For this review, take the finished solid that the model builds, in its own axes (mm). A direction names the side the tool comes from. Coordinates: 2 decimals unless noted, no trailing zeros. Order: outer loops, then holes, each group sorted by start corner. A loop starts at its lowest first (then second) coordinate and runs counter-clockwise, first axis right, second up. Notation, with made-up numbers: (-31.5, -5.75) - (17.5, -5.75) arc R15 cw to (17.5, 2.25) - close; hole circle Ø4 at (30, 14). An arc over 180 degrees is marked (long way). One line per item, written item: value. Start each with the question number.
(1) To check wall thickness, follow line 1 along Z through (x, y) = (0, 1.25); line 2 along Y through (x, z) = (4, -5.5); line 3 along Y through (x, z) = (13, -10.5). State the ranges of each line that lie inside material, in increasing order.
(2) Clearance check with flat-ended pins moving along their axes: pin 1 (4 mm diameter, centred on x = 8.5, y = 20.5, fed in from -Z); pin 2 (3 mm diameter, centred on x = -19.5, z = 7.5, fed in from +Y); pin 3 (5 mm diameter, centred on y = 21.5, z = 7, fed in from -X); pin 4 (12 mm diameter, centred on x = 5.5, y = 9, fed in from +Z). State where each tip first meets the part, or that it passes through.
(3) Consider section D-D on y = 28.5. Write out the cut boundary in (x, z), then the cut area to 3 significant figures.
(4) Mouldability with a two-part tool opening along X and no side actions: class faces 4 (the flat face through (0, 35, 0)), 5 (the conical face through (0.13, 5.35, 14.54)), 6 (the cylindrical face through (-2.343, 33.493, 17.847)) as released by +X, released by -X, zero draft, split by the parting line, or undercut.
(5) For faces 1 (the cylindrical face through (0.71, 1.72, -19.21)), 2 (the cylindrical face through (-2.85, 4.49, 17.13)), 3 (the flat face through (0, 0, 0)), list the 3-axis set-ups (+Z, -Z, +X, -X, +Y, -Y) from which the entire face can be reached by the end or side of a thin tool; tool diameter is ignored.
(6) Consider section C-C on y = 12.5. Write out the cut boundary in (x, z).
(7) Consider section B-B on x = 0. Count the separate pieces of the cut face and the enclosed holes in it, then the cut area to 3 significant figures.
Autodesk Inventor part; units mm, degrees
ref_plane "YZ Plane" through (0, 0, 0) normal (1, 0, 0) x (0, 1, 0)
ref_plane "XZ Plane" through (0, 0, 0) normal (0, 1, 0) x (-1, 0, 0)
ref_plane "XY Plane" through (0, 0, 0) normal (0, 0, 1) x (1, 0, 0)
sketch "Sketch2" plane through (0, 0, 0) normal (0, 0, 1) x (1, 0, 0)
  line L0 (0, 0) -> (25, 0)
  line L1 (0, 0) -> (0, 35)
  line L2 (0, 35) -> (18, 35)
  line L3 (18, 35) -> (18, 30)
  line L4 (18, 30) -> (5, 30)
  line L5 (5, 30) -> (5, 7)
  line L6 (5, 7) -> (25, 7)
  line L7 (25, 7) -> (25, 0)
  dimension "d3" = 25
  dimension "d4" = 35
  dimension "d5" = 18
  dimension "d6" = 5
  dimension "d23" = 7
  dimension "d24" = 23
  dimension "d26" = 5
revolve "Revolution1" add sketch "Sketch2" angle 360 about axis through (0, 0, 0) along (0, 1, 0)
fillet "Fillet1" radius 3 3 edges at (-5, 7, 0) (-18, 30, 0) (-25, 7, 0)
chamfer "Chamfer1" distance 1 angle 45 1 edges at (-18, 35, 0)
sketch "Sketch3" plane through (0, 0, 0) normal (0, -1, 0) x (1, 0, 0)
  line L0 (0, 0) -> (0, -17.5)
  line L1 (0, 0) -> (0, 17.5)
  dimension "d14" = 17.5
  dimension "d15" = 17.5
hole "Hole1" at (0, 0, 17.5) at (0, 0, -17.5) direction (0, 1, 0) diameter 3.7 depth 7
fillet "Fillet2" radius 10 1 edges at (-5, 30, 0)
sketch "Sketch4" plane through (0, 7, 0) normal (0, 1, 0) x (1, 0, 0)
  circle A0 centre (0, 17.5) radius 1.85
  circle A1 centre (0, -17.5) radius 1.85
  circle A2 centre (0, -17.5) radius 1.85
  circle A3 centre (0, -17.5) radius 1.85
  point P0 (0, 0)
hole "Hole2" at (0, 7, 17.5) at (0, 7, -17.5) direction (0, -1, 0) diameter 5.75 depth 3 tip angle 118
chamfer "Chamfer2" distance 0.5 distance2 2 1 edges at (0, 7, 14.625) measured on face at (-6.4693, 7, 13.5188)
chamfer "Chamfer3" distance 0.5 distance2 2 1 edges at (0, 7, -20.375) measured on face at (6.4693, 7, -13.5188)
sketch "Sketch5" plane through (0, 0, 0) normal (0, -1, 0) x (1, 0, 0)
  line L0 (-10, -10) -> (-10, 10)
  line L1 (-10, 10) -> (10, 10)
  line L2 (10, 10) -> (10, -10)
  line L3 (10, -10) -> (-10, -10)
  line L4 (-10, -10) -> (10, 10) construction
  line L5 (-10, 10) -> (10, -10) construction
  point P0 (0, 0)
  dimension "d34" = 20
  dimension "d35" = 20
extrude "Extrusion2" [suppressed]
sketch "Sketch7" plane through (0, 0, 0) normal (0, -1, 0) x (1, 0, 0)
  line L0 (-26, -7.75) -> (-10, -7.75)
  line L1 (-10, -7.75) -> (-10, 7.75)
  line L2 (-10, 7.75) -> (-26, 7.75)
  line L3 (-26, 7.75) -> (-26, -7.75)
  circle A0 centre (0, 0) radius 18
  line L4 (-26, -7.75) -> (-10, 7.75) construction
  line L5 (-10, -7.75) -> (-26, 7.75) construction
  point P0 (-18, 0)
  dimension "d44" = 15.5
extrude "Extrusion3" [suppressed]
sketch "Sketch8" plane through (-10, 0, 10) normal (0, -1, 0) x (1, 0, 0)
  arc A0 (35, -10) -> (35, -10) centre (10, -10) ccw
  line L0 (-12.5073, 0.8822) -> (-22.2437, 0.8822)
  line L1 (-22.2437, 0.8822) -> (-22.2437, -21.0128)
  line L2 (-22.2437, -21.0128) -> (-12.5073, -21.0128)
  line L3 (-12.5073, -21.0128) -> (-12.4075, -21.0862)
  arc A1 (-12.5073, 0.8822) -> (-12.4075, -21.0862) centre (10, -10) ccw
  point P0 (-13.7684, -17.75)
  point P1 (-13.7684, -2.25)
extrude "Extrusion4" [suppressed]
chamfer "Chamfer4" [suppressed]
fillet "Fillet3" [suppressed]
properties part number "holding_socket"
Geometry check:
1. line 1: z = -25 to -19.35, -15.65 to 15.65, 19.35 to 25
1. line 2: y = 0 to 7.25, 25.72 to 35
1. line 3: y = 0 to 7, 30.54 to 35
2. pin 1: passes through
2. pin 2: stops at y = 7
2. pin 3: stops at x = -2.52
2. pin 4: stops at z = 24.92
3. outline: circle Ø19.46 at (0, 0)
3. area: 298 mm^2
4. face 4: zero draft
4. face 5: undercut
4. face 6: split by the parting line
5. face 1: -Y
5. face 2: none
5. face 3: +Z, -Z, +X, -X, -Y
6. outline: circle Ø10 at (0, 0)
7. separate pieces: 3
7. enclosed holes: 0
7. area: 731 mm^2
